The drawing under review shows one solid part. Ordinate dimensions are in mm from its lowest x, y, z. A direction names the side the tool comes from. Give positions to 0.01 mm unless a question says otherwise; leave off trailing zeros. Write each loop counter-clockwise with the first axis right and the second up, starting at its lowest first coordinate (ties: lowest second). Pieces come first, ordered by that corner, then holes.
Q1. Insertion check: P1, Ø14.5, axis at y = 27, z = 27, coming from the +X side; P2, Ø2, axis at x = 5, z = 20.5, coming from the -Y side; P3, Ø3, axis at x = 12.5, z = 16, coming from the +Y side. Each pin has a flat end and moves straight along its axis. Give the tip position at first contact, or say it passes through.
Q2. Mouldability with a two-part tool opening along Y and no side actions: class the marked faces 1, 2 and 3 as released by +Y, released by -Y, zero draft, split by the parting line, or undercut.
Q3. Machinability: for the marked faces 4, 5 and 6, which of the approach directions +Z, -Z, +X, -X, +Y, -Y give a long, thin tool a straight path to every point of the face, cutting with its end or side? Answer none if there is none.
Q4. We need section D-D (y = 11.5). Write out the cut boundary in (x, z).
Q5. We need section A-A (z = 27). Write out the cut boundary in (x, y).
Q6. For line 1 (Y direction, x = 18, z = 27); line 2 (X direction, y = 33, z = 33.5); line 3 (Z direction, x = 18.5, y = 24), list the stretches that pass through material, from the lowest coordinate up.
Q7. We need section C-C (x = 13.75). Write out the cut boundary in (y, z), then the cut area to 3 significant figures.
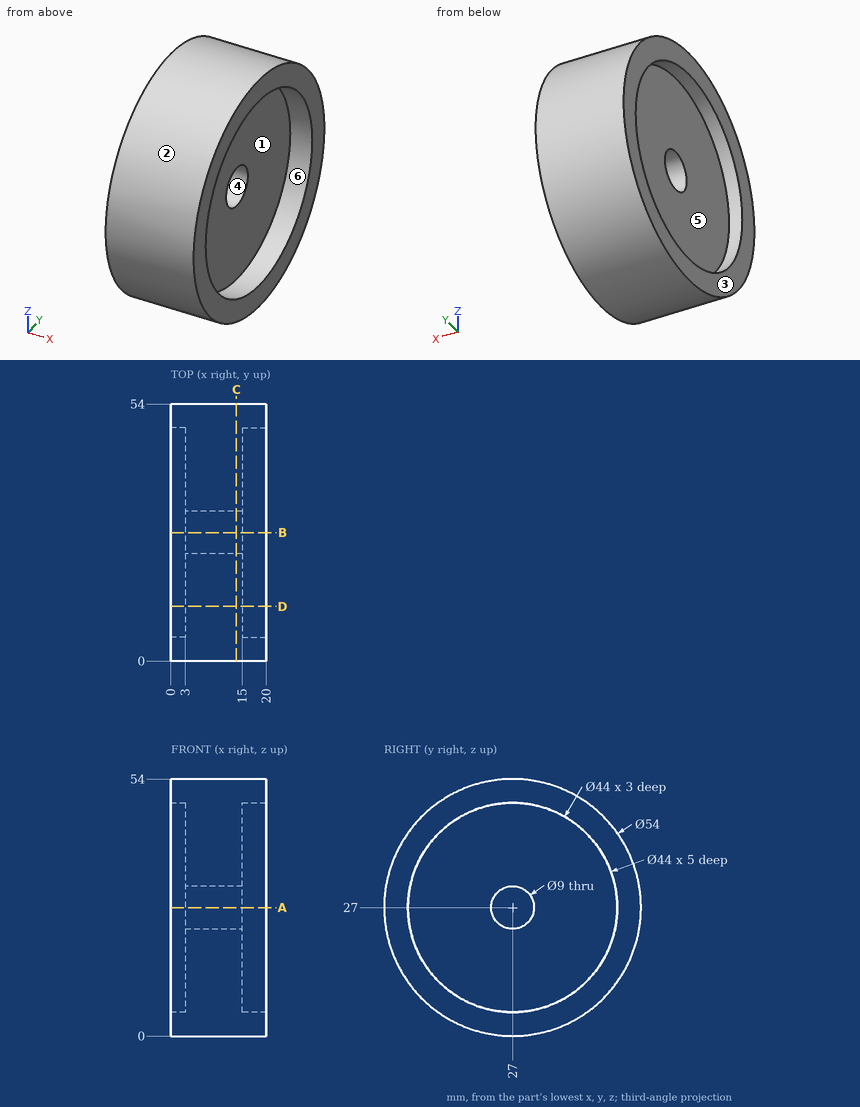
Computed:
1. P1: stops at x = 15
1. P2: stops at y = 0.57
1. P3: stops at y = 52.27
2. face 1: undercut
2. face 2: split by the parting line
2. face 3: zero draft
3. face 4: +X, -X
3. face 5: -X
3. face 6: +X
4. outline: (0, 4.89) - (20, 4.89) - (20, 11.39) - (15, 11.39) - (15, 42.61) - (20, 42.61) - (20, 49.11) - (0, 49.11) - (0, 42.61) - (3, 42.61) - (3, 11.39) - (0, 11.39) - close
5. outline: (0, 0) - (20, 0) - (20, 5) - (15, 5) - (15, 22.5) - (3, 22.5) - (3, 5) - (0, 5) - close; (0, 49) - (3, 49) - (3, 31.5) - (15, 31.5) - (15, 49) - (20, 49) - (20, 54) - (0, 54) - close
6. line 1: y = 0 to 5, 49 to 54
6. line 2: x = 3 to 15
6. line 3: z = 0.17 to 5.21, 48.79 to 53.83
7. outline: circle Ø54 at (27, 27); hole circle Ø9 at (27, 27)
7. area: 2,230 mm2
